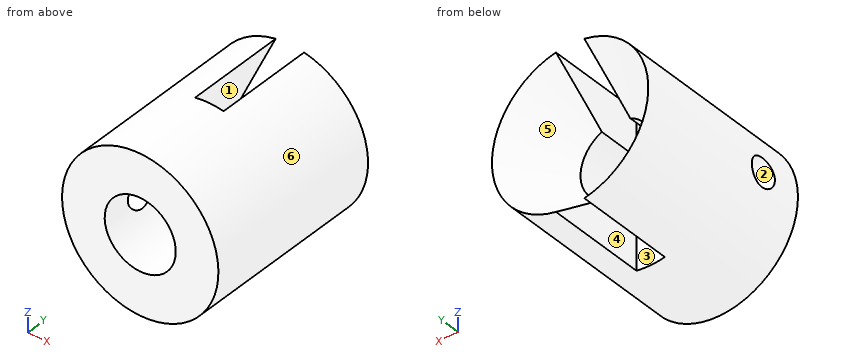
```python
from build123d import *

# Parameters (mm, degrees)
SKETCH1_R           = 5.5
BOSS_EXTRUDE1_DEPTH = 13
SKETCH2_R           = 2.5
CUT_EXTRUDE1_DEPTH  = 16.149257408
CHAMFER1_SIZE       = 3.0142162
CHAMFER1_SIZE_2     = 4
SKETCH4_W           = 2
SKETCH4_H           = 12
CUT_EXTRUDE2_DEPTH  = 7
SKETCH5_R           = 1
CUT_EXTRUDE3_DEPTH  = 7


with BuildPart() as part:
    # Sketch1 → Boss-Extrude1 (new body)
    with BuildSketch(Plane(origin=(0, 0, 0), x_dir=(1, 0, 0), z_dir=(0, 1, 0))):
        with Locations(Location((0, 0, 0), (0, 0, 90))):
            Circle(SKETCH1_R)
    extrude(amount=BOSS_EXTRUDE1_DEPTH)

    # Sketch2 → Cut-Extrude1 (cut, through all)
    with BuildSketch(Plane.XZ):
        with Locations(Location((0, 0, 0), (0, 0, 270))):
            Circle(SKETCH2_R)
    extrude(amount=-CUT_EXTRUDE1_DEPTH, mode=Mode.SUBTRACT)

    # Chamfer1
    # the kernel refuses this chamfer: 4, 3.0142162 mm, written as the material it takes off along each edge
    with BuildSketch(Plane(origin=(0, 13, 0), x_dir=(0, 0, -1), z_dir=(-1, 0, 0))) as chamfer1_piece_1:
        Polygon((2.5 + CHAMFER1_SIZE, 0), (2.5, CHAMFER1_SIZE_2), (2.5, 0), align=None)
    revolve(axis=Axis((0, 13, 0), (0, -1, 0)), mode=Mode.SUBTRACT)

    # Sketch4 → Cut-Extrude2 (cut)
    with BuildSketch(Plane(origin=(0, 13, 0), x_dir=(1, 0, 0), z_dir=(0, 1, 0))):
        Rectangle(SKETCH4_W, SKETCH4_H)
    extrude(amount=-CUT_EXTRUDE2_DEPTH, mode=Mode.SUBTRACT)

    # Sketch5 → Cut-Extrude3 (cut)
    with BuildSketch(Plane(origin=(0, 0, 0), x_dir=(0, 0, -1), z_dir=(1, 0, 0))):
        with Locations((0, 3)):
            Circle(SKETCH5_R)
    extrude(amount=-CUT_EXTRUDE3_DEPTH, mode=Mode.SUBTRACT)


solid = part.part
```
For this review, take the finished solid that the model builds, in its own axes (mm). Face numbers are marked on the shaded views. A direction names the side the tool comes from. Round coordinates to 2 decimals unless told otherwise and drop trailing zeros. Write each loop counter-clockwise with the first axis right and the second up, starting at its lowest first coordinate (ties: lowest second). Pieces come first, ordered by that corner, then holes.
1) For line 1 along Z through (x, y) = (-1, 1); line 2 along X through (y, z) = (6.75, 0); line 3 along X through (y, z) = (3.5, 0), list the stretches that pass through material, from the lowest coordinate up.
Answer below:
line 1: z = -5.41 to -2.29, 2.29 to 5.41
line 2: x = -5.5 to -2.5, 2.5 to 5.5
line 3: x = 2.5 to 5.5
2) Take a section at D-D on y = 3. Give the boundary of the cut face in (x, z).
Answer below:
outline: (-5.41, -1) arc R5.5 ccw (long way) to (-5.41, 1) - (-2.29, 1) arc R2.5 cw (long way) to (-2.29, -1) - close
3) Take a section at C-C on y = 11. Give the boundary of the cut face in (x, z).
Answer below:
outline: (-1, -5.41) - (-1, -3.88) arc R4.01 cw to (-1, 3.88) - (-1, 5.41) arc R5.5 ccw to start; (1, -5.41) arc R5.5 ccw to (1, 5.41) - (1, 3.88) arc R4.01 cw to (1, -3.88) - close
4) Mouldability with a two-part tool opening along Y and no side actions: class the marked faces 1, 2 and 3 as +Y half, -Y half, draft (parallel to the pull), parting line (faces both ways), or undercut.
Answer below:
face 1: draft
face 2: undercut
face 3: +Y half
5) Take a section at A-A on x = 0. Give the boundary of the cut face in (y, z), then the cut area to 3 significant figures.
Answer below:
outline: (0, -5.5) - (6, -5.5) - (6, -2.5) - (0, -2.5) - close; (0, 2.5) - (6, 2.5) - (6, 5.5) - (0, 5.5) - close
area: 36.0 mm2
6) Take a section at B-B on z = 0. Give the boundary of the cut face in (x, y).
Answer below:
outline: (-5.5, 0) - (-2.5, 0) - (-2.5, 2) - (-5.5, 2) - close; (-5.5, 4) - (-2.5, 4) - (-2.5, 9) - (-5.5, 12.98) - close; (2.5, 0) - (5.5, 0) - (5.5, 12.98) - (2.5, 9) - close
7) Insertion check: pin 1 Ø1 at (x, z) = (2.5, -1.5) entering from +Y; pin 2 Ø2 at (y, z) = (8, -1.5) entering from +X; pin 3 Ø1.6 at (y, z) = (9, -4) entering from +X. Each pin has a flat end and moves straight along its axis. Give the tip position at first contact, or say it passes through.
Answer below:
pin 1: stops at y = 10.21
pin 2: stops at x = 5.48
pin 3: stops at x = 4.47
8) Machinability: for the marked faces 4, 5 and 6, which of the approach directions +Z, -Z, +X, -X, +Y, -Y give a long, thin tool a straight path to every point of the face, cutting with its end or side? Answer none if there is none.
Answer below:
face 4: +Z, -Z, +Y
face 5: +Y
face 6: +Y, -Y
